from build123d import *

# Parameters (mm, degrees)
EXTRUDE_1_DEPTH      = 1
SKETCH_2_W           = 7
SKETCH_2_H           = 1
EXTRUDE_2_DEPTH      = 6
EXTRUDE_2_DEPTH_BACK = 6
FILLET_1_R           = 3
SKETCH_3_R           = 0.35
CUT_EXTRUDE_1_DEPTH  = 25.5
SKETCH_4_W           = 1
SKETCH_4_H           = 5
EXTRUDE_3_DEPTH      = 5
EXTRUDE_4_DEPTH      = 7
CUT_EXTRUDE_2_DEPTH  = 7


with BuildPart() as part:
    # 草图1 → 凸台-拉伸1 (new body)
    with BuildSketch(Plane(origin=(0, 0, 0), x_dir=(1, 0, 0), z_dir=(0, 1, 0))):
        Polygon((-12.5, 12.25), (11.2, 12.25), (11.2, -12.25), (-12.5, -12.25), (-19.5, -12.25), (-19.5, -11.25), (-12.5, -11.25), (-12.5, -5), (-19.5, -5), (-19.5, 5), (-12.5, 5), (-12.5, 11.25), (-19.5, 11.25), (-19.5, 12.25), align=None)
    extrude(amount=EXTRUDE_1_DEPTH)

    # 草图2 → 凸台-拉伸2 (add, two sides)
    with BuildSketch(Plane.XZ) as extrude_2_sk:
        with Locations((-16, 11.75)):
            Rectangle(SKETCH_2_W, SKETCH_2_H)
        with Locations((-16, -11.75)):
            Rectangle(SKETCH_2_W, SKETCH_2_H)
    extrude(amount=EXTRUDE_2_DEPTH)
    extrude(extrude_2_sk.sketch, amount=-EXTRUDE_2_DEPTH_BACK)

    # 圆角1
    fillet_1_edges = [part.edges().sort_by_distance(p)[0] for p in [
        (-19.5, 6, 11.75),
        (-19.5, 6, -11.75),
    ]]
    fillet(fillet_1_edges, radius=FILLET_1_R)

    # 草图3 → 切除-拉伸1 (cut, through all)
    with BuildSketch(Plane.XY.offset(12.25)):
        with Locations((-17.5, 0.5)):
            Circle(SKETCH_3_R)
        with Locations((-13.5, 5)):
            Circle(SKETCH_3_R)
    extrude(amount=-CUT_EXTRUDE_1_DEPTH, mode=Mode.SUBTRACT)

    # 草图4 → 凸台-拉伸3 (add)
    with BuildSketch(Plane(origin=(-12.5, 0, 0), x_dir=(0, 0, -1), z_dir=(1, 0, 0))):
        with Locations((-11.75, 3.5)):
            Rectangle(SKETCH_4_W, SKETCH_4_H)
        with Locations((11.75, 3.5)):
            Rectangle(SKETCH_4_W, SKETCH_4_H)
    extrude(amount=EXTRUDE_3_DEPTH)

    # 草图5 → 凸台-拉伸4 (add)
    with BuildSketch(Plane(origin=(0, 1, 0), x_dir=(1, 0, 0), z_dir=(0, 1, 0))):
        Polygon((-8.5, -8.25), (-8.5, -10.25), (5.5, -10.25), (5.5, -8.25), (4.5, -8.25), (4.5, -9.25), (-7.5, -9.25), (-7.5, -8.25), (-7.5, -3.5), (-7.5, -2.5), (2.5, -2.5), (2.5, -1.5), (-7.5, -1.5), (-7.5, 1.5), (2.5, 1.5), (2.5, 2.5), (-7.5, 2.5), (-7.5, 3.5), (-7.5, 8.25), (-7.5, 9.25), (4.5, 9.25), (4.5, 8.25), (5.5, 8.25), (5.5, 10.25), (-8.5, 10.25), (-8.5, 8.25), (-8.5, 3.742436738), (-8.5, 0.5), (-14.5, 0.5), (-14.5, -0.5), (-8.5, -0.5), (-8.5, -3.5), align=None)
    extrude(amount=EXTRUDE_4_DEPTH)

    # 草图6 → 切除-拉伸2 (cut)
    with BuildSketch(Plane.ZY.offset(8.5)):
        with BuildLine():
            Line((-8.25, 6.5), (-8.25, 9.621499742))
            Line((-8.25, 9.621499742), (-3.25, 9.621499742))
            Line((-3.25, 9.621499742), (-3.25, 6.5))
            ThreePointArc((-3.25, 6.5), (-5.75, 4), (-8.25, 6.5))
        make_face()
        with BuildLine():
            Line((3.25, 6.5), (3.25, 9.830182827))
            Line((3.25, 9.830182827), (8.25, 9.830182827))
            Line((8.25, 9.830182827), (8.25, 6.5))
            ThreePointArc((8.25, 6.5), (5.75, 4), (3.25, 6.5))
        make_face()
    extrude(amount=-CUT_EXTRUDE_2_DEPTH, mode=Mode.SUBTRACT)


solid = part.part
CAD build for the part. Positions are in the model's coordinates, mm. A direction names the side the tool comes from. Round coordinates to 2 decimals unless told otherwise and drop trailing zeros. Write each loop counter-clockwise with the first axis right and the second up, starting at its lowest first coordinate (ties: lowest second). Pieces come first, ordered by that corner, then holes. Notation, with made-up numbers: M -26,47 L 31,47 A7 ccw 31,60 Z; hole C -34.5,-20.75 d9. An arc over 180 degrees is marked long. Use a Markdown table: item, result. Add a question column.
1. 3-axis set-ups, long thin cutter, end or side, ignore diameter. For faces 4 (the face through (-19.5, 0.5, 0.1)), 5 (the face through (5, 4, 8.25)), 6 (the face through (-8.5, 3.7, -5.4)), 7 (the face through (-16, 0.5, -5)), 8 (the face through (-12.5, -3, 12)): which of +Z, -Z, +X, -X, +Y, -Y reach the whole face in a straight line?
2. Flat gauge pins, fed straight in: P1, Ø0.9, axis at y = 3, z = 0.5, coming from the +X side; P2, Ø0.8, axis at y = 3, z = 0, coming from the -X side; P3, Ø0.8, axis at x = 5, y = 5.5, coming from the -Z side. Where does each tip first touch, or does it go through?
3. Pull direction Z, two halves, no side cores. Call faces 1 (the face through (-12, 1, -12.25)), 2 (the face through (-2, 4, -9.25)), 3 (the face through (5.5, 4, 9)): released by +Z, released by -Z, zero draft, split by the parting line, or undercut.
4. Slice it at A-A on y = -2.5. Give the cut face in (x, z), then the cut area to 3 significant figures.
5. Slice it at C-C on x = -13.5. Give the cut face in (y, z).
6. Drill centre lines: probe 1 along Z at (x, y) = (1.5, 3); probe 2 along Z at (x, y) = (-16, 0.5); probe 3 along Y at (x, z) = (-13.5, 11.8). Where is each one in solid material? Low to high.
7. Slice it at D-D on y = 2. Give the number of separate pieces and of enclosed holes in the cut face, then the cut area to 3 significant figures.
8. Slice it at B-B on y = 0.5. Give the cut face in (x, z).
Reply:
| question | item | result |
|---|---|---|
| 1 | face 4 | +Z, -Z, -X, +Y, -Y |
| 1 | face 5 | +X, +Y |
| 1 | face 6 | -X, +Y |
| 1 | face 7 | -X, +Y, -Y |
| 1 | face 8 | +Z, -Z, +X, -Y |
| 2 | P1 | stops at x = -7.5 |
| 2 | P2 | stops at x = -14.5 |
| 2 | P3 | stops at z = -10.25 |
| 3 | face 1 | released by -Z |
| 3 | face 2 | undercut |
| 3 | face 3 | zero draft |
| 4 | outline | M -19.5,-12.25 L -12.5,-12.25 L -12.5,-11.25 L -19.5,-11.25 Z; M -19.5,11.25 L -12.5,11.25 L -12.5,12.25 L -19.5,12.25 Z |
| 4 | area | 14.0 mm^2 |
| 5 | outline | M -6,-12.25 L 4.65,-12.25 L 4.65,-11.25 L -6,-11.25 Z; M -6,11.25 L 4.65,11.25 L 4.65,12.25 L -6,12.25 Z; M 0,-5 L 1,-5 L 1,-0.5 L 8,-0.5 L 8,0.5 L 1,0.5 L 1,5 L 0,5 Z; M 5.35,-12.25 L 6,-12.25 L 6,-11.25 L 5.35,-11.25 Z; M 5.35,11.25 L 6,11.25 L 6,12.25 L 5.35,12.25 Z |
| 6 | probe 1 | z = -10.25 to -9.25, -2.5 to -1.5, 1.5 to 2.5, 9.25 to 10.25 |
| 6 | probe 2 | z = -12.25 to -11.25, -5 to 5, 11.25 to 12.25 |
| 6 | probe 3 | y = -6 to 4.65, 5.35 to 6 |
| 7 | separate pieces | 3 |
| 7 | enclosed holes | 0 |
| 7 | area | 98.5 mm^2 |
| 8 | outline | M -19.5,-12.25 L -17.85,-12.25 L -17.85,-11.25 L -19.5,-11.25 Z; M -19.5,-5 L -17.85,-5 L -17.85,5 L -19.5,5 Z; M -19.5,11.25 L -17.85,11.25 L -17.85,12.25 L -19.5,12.25 Z; M -17.15,-12.25 L 11.2,-12.25 L 11.2,12.25 L -17.15,12.25 L -17.15,11.25 L -12.5,11.25 L -12.5,5 L -17.15,5 L -17.15,-5 L -12.5,-5 L -12.5,-11.25 L -17.15,-11.25 Z |
